Geometry: final body of the model. Coordinates: model frame, mm. Coordinates: 2 decimals unless noted, no trailing zeros. Write each loop counter-clockwise with the first axis right and the second up, starting at its lowest first coordinate (ties: lowest second). Pieces come first, ordered by that corner, then holes. Notation, with made-up numbers: (64.5, 78) -> (81.5, 78) arc R15 cw to (81.5, 82) -> close; hole circle Ø10 at (43, 61.25). An arc over 180 degrees is marked (long way). Answer as a JSON object with one key per item and string values. Group by question number.
```python
from build123d import *

# Parameters (mm, degrees)
BOSS_EXTRUDE1_DEPTH = 3
FILLET1_R           = 4
FILLET2_R           = 3
FILLET3_R           = 1
FILLET5_R           = 0.5
SKETCH1_R           = 1
CUT_EXTRUDE1_DEPTH  = 2


with BuildPart() as part:
    # cover_itself → Boss-Extrude1 (new body)
    with BuildSketch(Plane(origin=(0, 0, 0), x_dir=(1, 0, 0), z_dir=(0, 1, 0))):
        with BuildLine():
            Line((-8.997858244, -0.196333965), (-10.480917414, 67.771305568))
            ThreePointArc((-10.480917414, 67.771305568), (-5.982302771, 76.608947935), (3.869342172, 77.743209027))
            Line((3.869342172, 77.743209027), (3.869342172, 43.384098405))
            Line((3.869342172, 43.384098405), (9.869342172, 39.743209027))
            Line((9.869342172, 39.743209027), (8.997858244, -0.196333965))
            ThreePointArc((8.997858244, -0.196333965), (0, -9), (-8.997858244, -0.196333965))
        make_face()
    extrude(amount=BOSS_EXTRUDE1_DEPTH)

    # Fillet1
    fillet1_edges = [part.edges().sort_by_distance(p)[0] for p in [
        (3.869342172, 1.5, -43.384098405),
    ]]
    fillet(fillet1_edges, radius=FILLET1_R)

    # Fillet2
    fillet2_edges = [part.edges().sort_by_distance(p)[0] for p in [
        (3.869342172, 1.5, -77.743209027),
    ]]
    fillet(fillet2_edges, radius=FILLET2_R)

    # Fillet3
    fillet3_edges = [part.edges().sort_by_distance(p)[0] for p in [
        (9.869342172, 1.5, -39.743209027),
    ]]
    fillet(fillet3_edges, radius=FILLET3_R)

    # Fillet5
    fillet5_edges = [part.edges().sort_by_distance(p)[0] for p in [
        (-9.739387829, 3, -33.787485802),
        (3.869342172, 3, -60.534214462),
        (4.383630471, 3, -43.673589393),
        (-7.054041855, 3, -75.755154705),
        (3.110493996, 3, -77.427046765),
        (7.585003856, 3, -41.129379545),
        (9.733712071, 3, -39.668799805),
        (0, 3, 9),
        (9.427302793, 3, -19.484831093),
    ]]
    fillet(fillet5_edges, radius=FILLET5_R)

    # Sketch1 → Cut-Extrude1 (cut)
    with BuildSketch(Plane.XZ):
        with Locations((-2.705062156, -1.67)):
            Circle(SKETCH1_R)
        with Locations((6.76984482, -35.216036183)):
            Circle(SKETCH1_R)
        with Locations((-5.399070001, -69.616613762)):
            Circle(SKETCH1_R)
    extrude(amount=-CUT_EXTRUDE1_DEPTH, mode=Mode.SUBTRACT)


solid = part.part
```
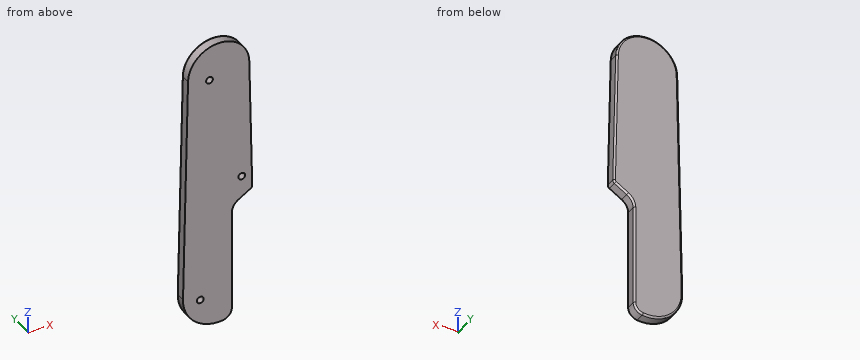
Item 1: Section A-A on y = 0.7. Output: boundary loops of the cut face in (x, z).
Item 2: Contact query for a flat-ended pin moving along its axis: pin 1 (0.6 mm diameter, centred on x = -5.5, z = -69.5, fed in from -Y). Output: stop coordinate, or through.
Item 3: Ray query, L1, parallel to X at y = 0.5, z = -67; L2, parallel to Z at x = 6.75, y = 1.25; L3, parallel to Z at x = 7.5, y = 0.7. Return the intervals inside material, ascending. Write a range as [from, to].
Answer sheet:
{
 "1": {"outline": "(-10.48, -67.77) arc R10.48 ccw to (1.22, -78.41) arc R3 ccw to (3.87, -75.43) -> (3.87, -45.64) arc R4 cw to (5.79, -42.22) -> (9.38, -40.04) arc R1 ccw to (9.86, -39.17) -> (9, 0.2) arc R9 ccw to (-9, 0.2) -> close; hole circle Ø2 at (-5.4, -69.62); hole circle Ø2 at (-2.71, -1.67); hole circle Ø2 at (6.77, -35.22)"},
 "2": {"pin 1": "stops at y = 2"},
 "3": {"L1": "x = [-10.46, 3.87]", "L2": "z = [-41.64, -36.22], [-34.22, 5.95]", "L3": "z = [-41.18, -35.9], [-34.53, 4.97]"}
}
